Part model, mm, in its own coordinate system. A direction names the side the tool comes from. Round coordinates to 2 decimals unless told otherwise and drop trailing zeros. Order: outer loops, then holes, each group sorted by start corner. A loop starts at its lowest first (then second) coordinate and runs counter-clockwise, first axis right, second up. Notation, with made-up numbers: M 84,48.5 L 93,48.5 A24 cw 93,61.5 Z; hole C 15.25,-34.75 d7. An arc over 180 degrees is marked long. Write each question's results on one line, items separated by ' | '. Start each with the question number.
1. Band-saw the part on A-A, the plane z = 45. List the corners of the cut face in (x, y).
2. Which spindle directions (+Z, -Z, +X, -X, +Y, -Y) get a long thin tool onto all of the face, cutting with end or side? Do faces 4 (the face through (-164, -3, 35)), 5 (the face through (152, 0, 0)). Say none if no direction does.
3. Band-saw the part on B-B, the plane y = 0. List the corners of the cut face in (x, z).
4. Two-plate mould, pull along X, no slides. Class faces 1 (the face through (3.837, -0.098, 174.458)), 2 (the face through (-2, 7, 147)), 3 (the face through (161, -3, 35)): +X half, -X half, draft (parallel to the pull), parting line (faces both ways), or undercut.
5. Probe L1, parallel to X at y = 0.25, z = 24; L2, parallel to Y at x = 162, z = 39; L3, parallel to Y at x = -162, z = 18. List the from-to ranges inside material, lowest first. Write a range as [from, to].
6. Band-saw the part on C-C, the plane x = 0. List the corners of the cut face in (y, z).
7. Drop flat-ended pins along their axis: pin 1 Ø2.5 at (x, y) = (-164.5, 0.5) entering from +Z; pin 2 Ø7 at (x, y) = (-162.5, 0) entering from -Z; pin 3 Ø3 at (x, y) = (58, -0.5) entering from -Z; pin 4 Ø6 at (y, z) = (-1, 139) entering from -X. Give the stop position or say it passes through.
8. Band-saw the part on D-D, the plane z = 159. List the corners of the cut face in (x, y), then the cut area to 3 significant figures.
```python
from build123d import *
from build123d import SkipClean  # not in build123d's __all__

# Parameters (mm, degrees)
F1_DEPTH = 7
F2_DEPTH = 6
F4_R     = 4.5
F5_DEPTH = 119.501
F6_DEPTH = 20
F7_R     = 3
F8_DEPTH = 35.0010001


# Not quite as in the source:
# - after a boolean that leaves OpenCascade's solid faulty, fix() repairs it


with BuildPart() as f1:
    # F0 (on Front) → F1 (new body, symmetric)
    with BuildSketch(Plane.XZ):
        with BuildLine():
            Line((129.5, 0), (174.5, 0))
            ThreePointArc((174.5, 0), (0, 174.5), (-174.5, 0))
            Line((-174.5, 0), (-129.5, 0))
            ThreePointArc((-129.5, 0), (0, 129.5), (129.5, 0))
        make_face()
    extrude(amount=F1_DEPTH, both=True)

    # F0 (on Front) → F2 (join, symmetric)
    with BuildSketch(Plane.XZ):
        with BuildLine():
            Line((129.5, 0), (174.5, 0))
            ThreePointArc((174.5, 0), (0, 174.5), (-174.5, 0))
            Line((-174.5, 0), (-129.5, 0))
            ThreePointArc((-129.5, 0), (0, 129.5), (129.5, 0))
        make_face()
    extrude(amount=F2_DEPTH, both=True)

    # F4 (on offset) → F5 (cut, through all)
    with BuildSketch(Plane.XY.offset(55)):
        with Locations((-162.5, 0)):
            Circle(F4_R)
        with Locations((162.5, 0)):
            Circle(F4_R)
    extrude(amount=F5_DEPTH, mode=Mode.SUBTRACT)

    # F4 (on offset) → F6 (cut)
    with BuildSketch(Plane.XY.offset(55)):
        with Locations((-162.5, 0)):
            Circle(F4_R)
        with Locations((162.5, 0)):
            Circle(F4_R)
    with SkipClean():  # cleaning this boolean's faces spoils the solid; the shape is the same uncleaned
        extrude(amount=-F6_DEPTH, mode=Mode.SUBTRACT)

    # F7 (on face) → F8 (cut, through all)
    with BuildSketch(Plane.XY.offset(35)):
        with Locations((-162.5, 0)):
            Circle(F7_R)
        with Locations((162.5, 0)):
            Circle(F7_R)
    extrude(amount=-F8_DEPTH, mode=Mode.SUBTRACT)

    add(f1.part.fix(), mode=Mode.REPLACE)


solid = f1.part
```
Solution:
1) outline: M -168.6,-7 L -121.43,-7 L -121.43,7 L -168.6,7 Z; M 121.43,-7 L 168.6,-7 L 168.6,7 L 121.43,7 Z; hole C -162.5,0 d9; hole C 162.5,0 d9
2) face 4: +Z | face 5: -Z, +X, -X, +Y, -Y
3) outline: M -174.5,0 L -165.5,0 L -165.5,35 L -167,35 L -167,50.61 A174.5 ccw Z; M -159.5,0 L -129.5,0 A129.5 cw 129.5,0 L 159.5,0 L 159.5,35 L 158,35 L 158,74.07 A174.5 ccw -158,74.07 L -158,35 L -159.5,35 Z; M 165.5,0 L 174.5,0 A174.5 ccw 167,50.61 L 167,35 L 165.5,35 Z
4) face 1: parting line | face 2: draft | face 3: undercut
5) L1: [-172.84, -165.49], [-159.51, -127.26], [127.26, 159.51], [165.49, 172.84] | L2: [-7, -4.47], [4.47, 7] | L3: [-7, -2.96], [2.96, 7]
6) outline: M -7,129.5 L 7,129.5 L 7,174.5 L -7,174.5 Z
7) pin 1: z = 35 | pin 2: z = 0 | pin 3: z = 115.02 | pin 4: x = -109.34
8) outline: M -71.9,-7 L 71.9,-7 L 71.9,7 L -71.9,7 Z | area: 2,010 mm^2
